Geometry check sheet. Reference: the model listing, model coordinates, mm. A direction names the side the tool comes from. Coordinates: 2 decimals unless noted, no trailing zeros. Write each loop counter-clockwise with the first axis right and the second up, starting at its lowest first coordinate (ties: lowest second). Pieces come first, ordered by that corner, then holes. Notation, with made-up numbers: M -39,72.5 L -23,72.5 A19 cw -23,107.5 Z; hole C 62,17 d7. An arc over 180 degrees is marked long. Answer as a JSON object with one key per item and string values. Group by question number.
```python
from build123d import *

# Parameters (mm, degrees)
ESBO_O1_R                = 1.6
ESBO_O1_W                = 28.5
ESBO_O1_H                = 10.6
ESBO_O1_W_2              = 30
ESBO_O1_H_2              = 69.1
ESBO_O1_W_3              = 20
ESBO_O1_H_3              = 4
RESSALTO_EXTRUS_O1_DEPTH = 6
FILETE3_R                = 3
FILETE4_R                = 10
FILETE5_R                = 7


with BuildPart() as part:
    # Esboço1 → Ressalto-extrusão1 (new body)
    with BuildSketch(Plane.XY):
        Polygon((-45.25, -56.75), (-23.05952475, -133.85), (23.05952475, -133.85), (45.25, -56.75), (45.25, 13.75), (57.5, 13.75), (57.5, 25.75), (45.25, 25.75), (45.25, 56.75), (16.663333, 56.75), (0, 73.75), (-16.663333, 56.75), (-45.25, 56.75), (-45.25, 25.75), (-57.5, 25.75), (-57.5, 13.75), (-45.25, 13.75), align=None)
        with Locations((0, 63.75)):
            Circle(ESBO_O1_R, mode=Mode.SUBTRACT)
        with Locations((-50.5, 20.75)):
            Circle(ESBO_O1_R, mode=Mode.SUBTRACT)
        with Locations((50.5, 20.75)):
            Circle(ESBO_O1_R, mode=Mode.SUBTRACT)
        with Locations((0, -118.55)):
            Rectangle(ESBO_O1_W, ESBO_O1_H, mode=Mode.SUBTRACT)
        with Locations((0, 7.2)):
            Rectangle(ESBO_O1_W_2, ESBO_O1_H_2, mode=Mode.SUBTRACT)
        with Locations((0, -54.75)):
            Rectangle(ESBO_O1_W_3, ESBO_O1_H_3, mode=Mode.SUBTRACT)
    extrude(amount=RESSALTO_EXTRUS_O1_DEPTH)

    # Filete3
    filete3_edges = [part.edges().sort_by_distance(p)[0] for p in [
        (-45.25, 13.75, 3),
        (45.25, 13.75, 3),
    ]]
    fillet(filete3_edges, radius=FILETE3_R)

    # Filete4
    filete4_edges = [part.edges().sort_by_distance(p)[0] for p in [
        (-45.25, 25.75, 3),
        (-45.25, 56.75, 3),
        (-16.663333, 56.75, 3),
        (0, 73.75, 3),
        (16.663333, 56.75, 3),
        (45.25, 56.75, 3),
        (45.25, 25.75, 3),
        (45.25, -56.75, 3),
        (23.05952475, -133.85, 3),
        (-23.05952475, -133.85, 3),
        (-45.25, -56.75, 3),
    ]]
    fillet(filete4_edges, radius=FILETE4_R)

    # Filete5
    # the kernel refuses this fillet: 7 mm, written as the material it adds along each edge
    with BuildSketch(Plane(origin=(-15, -27.35, 0), x_dir=(1, 0, 0), z_dir=(0, 0, 1)), Plane(origin=(15, 41.75, 0), x_dir=(-1, 0, 0), z_dir=(0, 0, 1)), Plane(origin=(-15, 41.75, 0), x_dir=(0, -1, 0), z_dir=(0, 0, 1))) as filete5_piece_1:
        with BuildLine():
            CenterArc((FILETE5_R, FILETE5_R), FILETE5_R, 180, 90)
            Line((0, FILETE5_R), (0, 0))
            Line((0, 0), (FILETE5_R, 0))
        make_face()
    extrude(amount=6)
    with BuildSketch(Plane(origin=(15, -27.35, 0), x_dir=(-1, 0, 0), z_dir=(0, 0, 1))) as filete5_piece_2:
        with BuildLine():
            CenterArc((FILETE5_R, -FILETE5_R), FILETE5_R, 90, 90)
            Line((0, -FILETE5_R), (0, 0))
            Line((0, 0), (FILETE5_R, 0))
        make_face()
    extrude(amount=6)
    # the kernel refuses this fillet: 7 mm, written as the material it takes off along each edge
    with BuildSketch(Plane(origin=(57.5, 13.75, -17.5), x_dir=(-1, 0, 0), z_dir=(0, 0, 1))) as filete5_2_piece_1:
        with BuildLine():
            CenterArc((FILETE5_R, -FILETE5_R), FILETE5_R, 90, 90)
            Line((0, -FILETE5_R), (0, 0))
            Line((0, 0), (FILETE5_R, 0))
        make_face()
    extrude(amount=41, mode=Mode.SUBTRACT)
    with BuildSketch(Plane(origin=(57.5, 25.75, -15.807283357), x_dir=(0, -1, 0), z_dir=(0, 0, 1))) as filete5_2_piece_2:
        with BuildLine():
            CenterArc((6.322913343, -7), FILETE5_R, 90, 73.774899865)
            Line((-0.398286269, -5.044117647), (-1.07040623, -4.848529412))
            ThreePointArc((-1.07040623, -4.848529412), (-0.7, -2.25), (-0.7, 0))
            Line((-0.7, 0), (0, 0.7))
            Line((0, 0.7), (6.322913343, 0.7))
            Line((6.322913343, 0.7), (6.322913343, 0))
        make_face()
    extrude(amount=37.614566715, mode=Mode.SUBTRACT)
    with BuildSketch(Plane(origin=(-57.5, 13.75, -17.5), x_dir=(1, 0, 0), z_dir=(0, 0, 1))) as filete5_2_piece_3:
        with BuildLine():
            CenterArc((FILETE5_R, FILETE5_R), FILETE5_R, 180, 90)
            Line((0, FILETE5_R), (0, 0))
            Line((0, 0), (FILETE5_R, 0))
        make_face()
    extrude(amount=41, mode=Mode.SUBTRACT)
    with BuildSketch(Plane(origin=(-57.5, 25.75, -15.807283357), x_dir=(0, -1, 0), z_dir=(0, 0, 1))) as filete5_2_piece_4:
        with BuildLine():
            CenterArc((6.322913343, 7), FILETE5_R, 196.225100135, 73.774899865)
            Line((-0.398286269, 5.044117647), (-1.07040623, 4.848529412))
            ThreePointArc((-1.07040623, 4.848529412), (-0.7, 2.25), (-0.7, 0))
            Line((-0.7, 0), (0, -0.7))
            Line((0, -0.7), (6.322913343, -0.7))
            Line((6.322913343, -0.7), (6.322913343, 0))
        make_face()
    extrude(amount=37.614566715, mode=Mode.SUBTRACT)


solid = part.part
```
1) Section check A-A (y = -10.5). Record the cut outline in (x, z).
2) Section check C-C (x = -32.5). Record the cut outline in (y, z), then the cut area to 3 significant figures.
3) Draft check along Y on faces 1 (the cylindrical face through (-55.26, 15.62, 2.96)), 2 (the cylindrical face through (16.94, 57.55, 3.04)), 3 (the flat face through (14.25, -119, 3)). Enter one of: +Y half, -Y half, draft (parallel to the pull), parting line (faces both ways), or undercut.
4) Section check B-B (z = 1.3). State how many separate pieces and enclosed holes the cut face has, then the cut area to 3 significant figures.
5) Material ranges on probe 1 along Y at (x, z) = (0, 3.3); probe 2 along X at (y, z) = (-7.5, 0.8); probe 3 along X at (y, z) = (-23, 3.95), recorded low to high. Write a range as [from, to].
6) Section check D-D (y = -83). Record the cut outline in (x, z).
7) Set-up check for faces 4 (the flat face through (0, -27.35, 3)), 5 (the flat face through (45.25, -23, 3)), 6 (the flat face through (45.25, 41, 3)): record each of +Z, -Z, +X, -X, +Y, -Y from which the full face is reachable in a straight line by a thin tool's end or side.
8) Go/stop test with flat-tipped pins: pin 1 Ø3 at (x, y) = (50.5, 20.75) entering from -Z; pin 2 Ø3 at (x, z) = (21.5, 4) entering from -Y; pin 3 Ø1.8 at (x, z) = (49, 2) entering from -Y; pin 4 Ø1.2 at (y, z) = (-55, 2) entering from +X. Record where each tip stops, or that it passes through.
Entries:
{
 "1": {"outline": "M -45.25,0 L -15,0 L -15,6 L -45.25,6 Z; M 15,0 L 45.25,0 L 45.25,6 L 15,6 Z"},
 "2": {"outline": "M -101.05,0 L 56.75,0 L 56.75,6 L -101.05,6 Z", "area": "947 mm^2"},
 "3": {"face 1": "-Y half", "face 2": "+Y half", "face 3": "undercut"},
 "4": {"separate pieces": "1", "enclosed holes": "6", "area": "13,600 mm^2"},
 "5": {"probe 1": "[-133.85, -123.85], [-113.25, -56.75], [-52.75, -27.35], [41.75, 62.15], [65.35, 69.46]", "probe 2": "[-45.25, -15], [15, 45.25]", "probe 3": "[-45.25, -14.48], [14.48, 45.25]"},
 "6": {"outline": "M -37.69,0 L 37.69,0 L 37.69,6 L -37.69,6 Z"},
 "7": {"face 4": "+Z, -Z", "face 5": "+Z, -Z, +X, -Y", "face 6": "+Z, -Z, +X, +Y"},
 "8": {"pin 1": "through", "pin 2": "y = -132.8", "pin 3": "y = 13.75", "pin 4": "x = 45.25"}
}
